```python
from build123d import *

# Parameters (mm, degrees)
SZKIC1_W                    = 137.1
SZKIC1_H                    = 80.8
DODANIE_WYCI_GNI_CIE1_DEPTH = 27.8
SZKIC2_W                    = 92.445066106
SZKIC2_H                    = 9.2
SZKIC2_W_2                  = 18.000987162
SZKIC2_H_2                  = 80.8
WYTNIJ_WYCI_GNI_CIE1_DEPTH  = 10
SZKIC3_R                    = 1.25
WYTNIJ_WYCI_GNI_CIE2_DEPTH  = 5


with BuildPart() as part:
    # Szkic1 → Dodanie-wyciągnięcie1 (new body)
    with BuildSketch(Plane.XY):
        with Locations((-7.480300087, -6.972885306)):
            Rectangle(SZKIC1_W, SZKIC1_H)
    extrude(amount=DODANIE_WYCI_GNI_CIE1_DEPTH)

    # Szkic2 → Wytnij-wyciągnięcie1 (cut)
    with BuildSketch(Plane.XY.offset(27.8)):
        with Locations((-20.948912207, -42.772885306)):
            Rectangle(SZKIC2_W, SZKIC2_H)
        with Locations((-20.948912207, 28.827114694)):
            Rectangle(SZKIC2_W, SZKIC2_H)
        with Locations((52.069206332, -6.972885306)):
            Rectangle(SZKIC2_W_2, SZKIC2_H_2)
    extrude(amount=-WYTNIJ_WYCI_GNI_CIE1_DEPTH, mode=Mode.SUBTRACT)

    # Szkic3 → Wytnij-wyciągnięcie2 (cut)
    with BuildSketch(Plane(origin=(0, 0, 0), x_dir=(-1, 0, 0), z_dir=(0, 0, -1))):
        with Locations((65.580300087, 12.777114694)):
            Circle(SZKIC3_R)
        with Locations((65.580300087, -26.722885306)):
            Circle(SZKIC3_R)
        with Locations((-35.819699913, -26.722885306)):
            Circle(SZKIC3_R)
        with Locations((-35.819699913, 14.027114694)):
            Circle(SZKIC3_R)
    extrude(amount=-WYTNIJ_WYCI_GNI_CIE2_DEPTH, mode=Mode.SUBTRACT)


solid = part.part
```
Check sheet for the modelled part. Datum: model origin and axes. Units: mm. A direction names the side the tool comes from. Round coordinates to 2 decimals unless told otherwise and drop trailing zeros. Order: outer loops, then holes, each group sorted by start corner. A loop starts at its lowest first (then second) coordinate and runs counter-clockwise, first axis right, second up. Notation, with made-up numbers: (-3.5, 69) - (4.5, 69) arc R11 ccw to (4.5, 88) - close; hole circle Ø6 at (30.25, -18). An arc over 180 degrees is marked (long way). Write item = value, one per line.
Q1. Section check C-C (x = -44). Record the boundary of the cut face in (y, z), and give its area (3 significant figures).
Computed:
outline = (-47.37, 0) - (33.43, 0) - (33.43, 17.8) - (24.23, 17.8) - (24.23, 27.8) - (-38.17, 27.8) - (-38.17, 17.8) - (-47.37, 17.8) - close
area = 2,060 mm^2
Q2. Section check D-D (y = -5). Record the boundary of the cut face in (x, z), and give its area (3 significant figures).
Computed:
outline = (-76.03, 0) - (61.07, 0) - (61.07, 17.8) - (43.07, 17.8) - (43.07, 27.8) - (-76.03, 27.8) - close
area = 3,630 mm^2
Q3. Draft check along Y on faces 1 (the face through (-22, 24.227, 23)), 2 (the face through (37.07, 14.08, 2.46)), 3 (the face through (-22, 29, 17.8)), 4 (the face through (-22, -38.173, 23)). Enter one of: pulls with the +Y half, pulls with the -Y half, needs draft (parallel to the pull), parting line crosses it, or undercut.
Computed:
face_1 = pulls with the +Y half
face_2 = undercut
face_3 = needs draft
face_4 = pulls with the -Y half
Q4. Section check B-B (z = 25.25). Record the boundary of the cut face in (x, y).
Computed:
outline = (-76.03, -47.37) - (-67.17, -47.37) - (-67.17, -38.17) - (25.27, -38.17) - (25.27, -47.37) - (43.07, -47.37) - (43.07, 33.43) - (25.27, 33.43) - (25.27, 24.23) - (-67.17, 24.23) - (-67.17, 33.43) - (-76.03, 33.43) - close
Q5. Section check A-A (y = 28). Record the boundary of the cut face in (x, z).
Computed:
outline = (-76.03, 0) - (61.07, 0) - (61.07, 17.8) - (43.07, 17.8) - (43.07, 27.8) - (25.27, 27.8) - (25.27, 17.8) - (-67.17, 17.8) - (-67.17, 27.8) - (-76.03, 27.8) - close
Q6. Tool access check on faces 5 (the face through (43.069, -8, 23)), 6 (the face through (-64.6, -27.5, 2.5)), 7 (the face through (-67.171, -43, 23)). Record the directions out of +Z, -Z, +X, -X, +Y, -Y that give a thin tool (end or side, any length) a straight path to the whole face; none if there is none.
Computed:
face_5 = +Z, +X, +Y, -Y
face_6 = -Z
face_7 = +Z, -Y
Q7. Go/stop test with flat-tipped pins: pin 1 (10 mm diameter, centred on x = 1, y = 30, fed in from +Z); pin 2 (4 mm diameter, centred on x = 16, z = 23.5, fed in from +Y); pin 3 (5 mm diameter, centred on y = -24, z = 22, fed in from +X). Record where each tip stops, or that it passes through.
Computed:
pin_1 = 17.8
pin_2 = 24.23
pin_3 = 43.07
Q8. Thickness scan on line 1 along X through (y, z) = (25.5, 19.5); line 2 along X through (y, z) = (-5.5, 20.75); line 3 along Z through (x, y) = (49.5, -18.5). Record the ranges inside material, lowest first.
Computed:
line_1 = -76.03 to -67.17, 25.27 to 43.07
line_2 = -76.03 to 43.07
line_3 = 0 to 17.8
